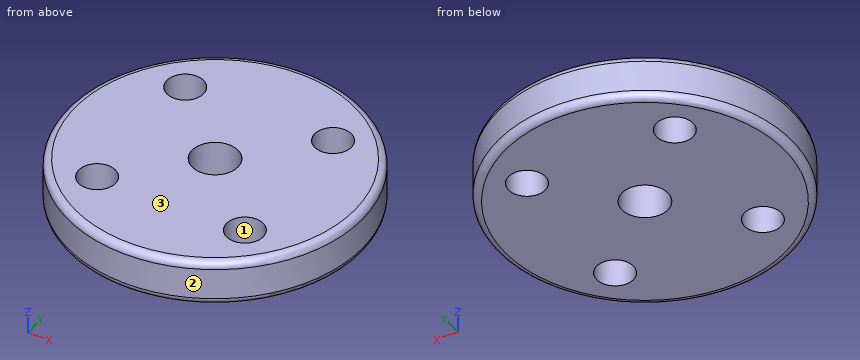
from build123d import *

# Parameters (mm, degrees)
SKETCH1_R      = 16
SKETCH1_R_2    = 2
SKETCH1_R_3    = 2.5
EXTRUDE2_DEPTH = 5
FILLET1_R      = 0.8


with BuildPart() as part:
    # Sketch1 → Extrude2 (new body)
    with BuildSketch(Plane.XY):
        Circle(SKETCH1_R)
        with Locations((-8, 8)):
            Circle(SKETCH1_R_2, mode=Mode.SUBTRACT)
        with Locations((-8, -8)):
            Circle(SKETCH1_R_2, mode=Mode.SUBTRACT)
        with Locations((8, -8)):
            Circle(SKETCH1_R_2, mode=Mode.SUBTRACT)
        with Locations((8, 8)):
            Circle(SKETCH1_R_2, mode=Mode.SUBTRACT)
        Circle(SKETCH1_R_3, mode=Mode.SUBTRACT)
    extrude(amount=EXTRUDE2_DEPTH)

    # Fillet1
    fillet1_edges = [part.edges().sort_by_distance(p)[0] for p in [
        (-16, 0, 5),
        (-16, 0, 0),
    ]]
    fillet(fillet1_edges, radius=FILLET1_R)


solid = part.part
Here's how the part is built. I have some questions about the finished solid (model axes, mm). Face numbers are marked on the shaded views. Round coordinates to 2 decimals unless told otherwise and drop trailing zeros. Write each loop counter-clockwise with the first axis right and the second up, starting at its lowest first coordinate (ties: lowest second). Pieces come first, ordered by that corner, then holes.
1. Suppose I cut it at D-D (y = -8). State how many separate pieces and enclosed holes the cut face has, and give its area (3 significant figures).
2. Suppose I cut it at A-A (x = 0). List the corners of the cut face in (y, z) for me, and give its area (3 significant figures).
3. Suppose I cut it at C-C (z = 3.75). List the corners of the cut face in (x, y) for me.
4. Will these pins go through, and if not, where does the flat tip stop? pin 1 Ø3 at (x, z) = (6.5, 2) entering from +Y; pin 2 Ø2 at (y, z) = (-7.5, 3) entering from +X; pin 3 Ø2 at (y, z) = (-5.5, 0.5) entering from -X.
5. I need wall thicknesses on L1, parallel to Y at x = 0, z = 2.8; L2, parallel to Y at x = -9.5, z = 1.75; L3, parallel to Y at x = -8, z = 1.3. Which ranges of each line are inside material? Lowest first, please.
6. If we mould it in two halves opening along Y, with no side actions, what happens to the marked faces 1, 2 and 3? For each: released by +Y, released by -Y, zero draft, split by the parting line, or undercut.
Answer sheet:
1. separate pieces: 3
1. enclosed holes: 0
1. area: 97.9 mm2
2. outline: (-16, 0.8) arc R0.8 ccw to (-15.2, 0) - (-2.5, 0) - (-2.5, 5) - (-15.2, 5) arc R0.8 ccw to (-16, 4.2) - close; (2.5, 0) - (15.2, 0) arc R0.8 ccw to (16, 0.8) - (16, 4.2) arc R0.8 ccw to (15.2, 5) - (2.5, 5) - close
2. area: 134 mm2
3. outline: circle Ø32 at (0, 0); hole circle Ø4 at (-8, -8); hole circle Ø4 at (-8, 8); hole circle Ø5 at (0, 0); hole circle Ø4 at (8, -8); hole circle Ø4 at (8, 8)
4. pin 1: stops at y = 15.2
4. pin 2: stops at x = 14.62
4. pin 3: stops at x = -15.34
5. L1: y = -16 to -2.5, 2.5 to 16
5. L2: y = -12.87 to -9.32, -6.68 to 6.68, 9.32 to 12.87
5. L3: y = -13.86 to -10, -6 to 6, 10 to 13.86
6. face 1: undercut
6. face 2: split by the parting line
6. face 3: zero draft
